Geometry: final body of the model. Coordinates: model frame, mm. A direction names the side the tool comes from. Give positions to 0.01 mm unless a question says otherwise; leave off trailing zeros. Order: outer loops, then holes, each group sorted by start corner. A loop starts at its lowest first (then second) coordinate and runs counter-clockwise, first axis right, second up. Notation, with made-up numbers: (-27.75, 49.5) - (16.25, 49.5) arc R9 ccw to (16.25, 61.5) - close; hole circle Ø8 at (8.5, 82.25). An arc over 180 degrees is marked (long way). One line per item, written item: value.
```python
from build123d import *

# Parameters (mm, degrees)
SKETCH1_R                     = 2.15265
SKETCH1_R_2                   = 9.525
BOSS_EXTRUDE1_DEPTH           = 1.5875
CUT_EXTRUDE1_DEPTH            = 2.54
F_13_64_0_18_DIAMETER_HOLE1_D = 4.572


with BuildPart() as part:
    # Sketch1 → Boss-Extrude1 (new body)
    with BuildSketch(Plane(origin=(0, 0, 0), x_dir=(1, 0, 0), z_dir=(0, 1, 0))):
        with BuildLine():
            Line((-107.315, 152.4), (-146.05, 152.4))
            Line((-146.05, 152.4), (-146.05, -152.4))
            Line((-146.05, -152.4), (146.05, -152.4))
            Line((146.05, -152.4), (146.05, 152.4))
            Line((146.05, 152.4), (107.315, 152.4))
            Line((107.315, 152.4), (107.315, 149.225))
            ThreePointArc((107.315, 149.225), (105.455128061, 144.734871939), (100.965, 142.875))
            Line((100.965, 142.875), (-100.965, 142.875))
            ThreePointArc((-100.965, 142.875), (-105.455128061, 144.734871939), (-107.315, 149.225))
            Line((-107.315, 149.225), (-107.315, 152.4))
        make_face()
        with Locations(Location((-135.128, -118.872, 0), (0, 0, 270))):
            Circle(SKETCH1_R, mode=Mode.SUBTRACT)
        with Locations(Location((-91.44, -91.44, 0), (0, 0, 270))):
            Circle(SKETCH1_R_2, mode=Mode.SUBTRACT)
        with Locations(Location((-113.665, -57.15, 0), (0, 0, 270))):
            Circle(SKETCH1_R, mode=Mode.SUBTRACT)
        with Locations(Location((-113.665, -38.1, 0), (0, 0, 270))):
            Circle(SKETCH1_R, mode=Mode.SUBTRACT)
        with Locations(Location((-91.44, -47.244, 0), (0, 0, 270))):
            Circle(SKETCH1_R_2, mode=Mode.SUBTRACT)
        with Locations(Location((-91.44, -3.048, 0), (0, 0, 270))):
            Circle(SKETCH1_R_2, mode=Mode.SUBTRACT)
        with BuildLine():
            ThreePointArc((-100.965, -117.475), (-107.315, -111.125), (-100.965, -104.775))
            Line((-100.965, -104.775), (100.965, -104.775))
            ThreePointArc((100.965, -104.775), (107.315, -111.125), (100.965, -117.475))
            Line((100.965, -117.475), (-100.965, -117.475))
        make_face(mode=Mode.SUBTRACT)
        with Locations(Location((135.128, -118.872, 0), (0, 0, 270))):
            Circle(SKETCH1_R, mode=Mode.SUBTRACT)
        with Locations(Location((91.44, -91.44, 0), (0, 0, 270))):
            Circle(SKETCH1_R_2, mode=Mode.SUBTRACT)
        with Locations(Location((91.44, -47.244, 0), (0, 0, 270))):
            Circle(SKETCH1_R_2, mode=Mode.SUBTRACT)
        with Locations(Location((113.665, -57.15, 0), (0, 0, 270))):
            Circle(SKETCH1_R, mode=Mode.SUBTRACT)
        with Locations(Location((113.665, -38.1, 0), (0, 0, 270))):
            Circle(SKETCH1_R, mode=Mode.SUBTRACT)
        with Locations(Location((91.44, -3.048, 0), (0, 0, 270))):
            Circle(SKETCH1_R_2, mode=Mode.SUBTRACT)
        with Locations(Location((-113.665, 76.2, 0), (0, 0, 270))):
            Circle(SKETCH1_R, mode=Mode.SUBTRACT)
        with Locations(Location((-91.44, 41.148, 0), (0, 0, 270))):
            Circle(SKETCH1_R_2, mode=Mode.SUBTRACT)
        with Locations(Location((-113.665, 95.25, 0), (0, 0, 270))):
            Circle(SKETCH1_R, mode=Mode.SUBTRACT)
        with Locations(Location((-91.44, 85.344, 0), (0, 0, 270))):
            Circle(SKETCH1_R_2, mode=Mode.SUBTRACT)
        with Locations(Location((-135.128, 141.478, 0), (0, 0, 270))):
            Circle(SKETCH1_R, mode=Mode.SUBTRACT)
        with Locations(Location((-91.44, 129.54, 0), (0, 0, 270))):
            Circle(SKETCH1_R_2, mode=Mode.SUBTRACT)
        with Locations(Location((91.44, 41.148, 0), (0, 0, 270))):
            Circle(SKETCH1_R_2, mode=Mode.SUBTRACT)
        with Locations(Location((113.665, 76.2, 0), (0, 0, 270))):
            Circle(SKETCH1_R, mode=Mode.SUBTRACT)
        with Locations(Location((91.44, 85.344, 0), (0, 0, 270))):
            Circle(SKETCH1_R_2, mode=Mode.SUBTRACT)
        with Locations(Location((113.665, 95.25, 0), (0, 0, 270))):
            Circle(SKETCH1_R, mode=Mode.SUBTRACT)
        with Locations(Location((91.44, 129.54, 0), (0, 0, 270))):
            Circle(SKETCH1_R_2, mode=Mode.SUBTRACT)
        with Locations(Location((135.128, 141.478, 0), (0, 0, 270))):
            Circle(SKETCH1_R, mode=Mode.SUBTRACT)
    extrude(amount=BOSS_EXTRUDE1_DEPTH)

    # Sketch2 → Cut-Extrude1 (cut)
    with BuildSketch(Plane(origin=(0, 1.5875, 0), x_dir=(1, 0, 0), z_dir=(0, 1, 0))):
        Polygon((-23.413358533, 142.875), (-29.763358533, 142.875), (-29.763358533, 116.18638997), (-29.763358533, 111.10638997), (-23.413358533, 111.10638997), (-10.745128401, 111.10638997), (-10.745128401, 80.773994761), (-10.745128401, 71.647772826), (-39.37, 71.647772826), (-39.37, 54.61788987), (-39.37, 43.18), (-33.02, 43.18), (-33.02, 54.61788987), (-33.02, 65.297772826), (-4.395128401, 65.297772826), (-4.395128401, 74.423994761), (-4.395128401, 82.043994761), (-4.395128401, 111.10638997), (-4.395128401, 117.45638997), (-23.413358533, 117.45638997), align=None)
        Polygon((51.818643407, 142.875), (45.468643407, 142.875), (45.468643407, 123.598152459), (26.196923788, 123.598152459), (26.196923788, 117.248152459), (26.196923788, 65.497956958), (50.548643407, 65.497956958), (50.548643407, 46.447956958), (26.196923788, 46.447956958), (25.908, -26.035), (32.258, -26.035), (32.258, -6.148708856), (32.258, -3.919741149), (32.258, 40.097956958), (56.898643407, 40.097956958), (56.898643407, 71.847956958), (32.546923788, 71.847956958), (32.546923788, 117.248152459), (51.818643407, 117.248152459), align=None)
    extrude(amount=-CUT_EXTRUDE1_DEPTH, mode=Mode.SUBTRACT)

    # 13/64 (0.18) Diameter Hole1 (through all)
    with Locations(Plane(origin=(0, 0, 0), x_dir=(-1, 0, 0), z_dir=(0, -1, 0))):
        with Locations((-57.15, 107.315), (-57.15, 84.455), (38.1, 84.455), (38.1, 107.315)):
            Hole(F_13_64_0_18_DIAMETER_HOLE1_D / 2)


solid = part.part
```
1) Mould query, pull axis Z, two halves, no side actions, for faces 4 (the face through (-2, 1.588, -2)), 5 (the face through (105.5, 0.78, -144.78)), 6 (the face through (107.313, 0.783, 110.985)). Classes: released by +Z, released by -Z, zero draft, split by the parting line, or undercut.
Answers below:
face 4: zero draft
face 5: released by -Z
face 6: undercut
2) Section A-A, the plane x = 17. Return loops of the section in (y, z) (1 decimal).
Answers below:
outline: (0, -142.9) - (1.6, -142.9) - (1.6, 104.8) - (0, 104.8) - close; (0, 117.5) - (1.6, 117.5) - (1.6, 152.4) - (0, 152.4) - close
3) First-contact query: pin 1 (0.8 mm diameter, centred on x = -81, y = 1, fed in from -Z) (3 decimals). Flat tip, straight axial feed; report the tip coordinate or a pass-through.
Answers below:
pin 1: z = -142.875
4) Material intervals for line 1 along Z through (x, y) = (-26, 0.5) (3 decimals); line 2 along X through (y, z) = (0.4, -61); line 3 along Z through (x, y) = (34, 1.55) (3 decimals), sorted ascending.
Answers below:
line 1: -111.106 to -71.648, -65.298 to 104.775, 117.475 to 152.4
line 2: -146.05 to -39.37, -33.02 to 50.55, 56.9 to 146.05
line 3: -142.875 to -123.598, -117.248 to -71.848, -65.498 to -46.448, -40.098 to 104.775, 117.475 to 152.4
5) Set-up query: faces 1 (the face through (-107.313, 0.783, 111.265)), 2 (the face through (-105.41, 0.78, -144.69)), 3 (the face through (-2, 0, -2)). Return all of +Z, -Z, +X, -X, +Y, -Y with unobstructed straight access to the full face (end or side cutting, diameter ignored); none if empty.
Answers below:
face 1: +Y, -Y
face 2: -Z, +Y, -Y
face 3: +Z, -Z, +X, -X, -Y
6) Section B-B, the plane z = 91.44. Count the separate pieces of the cut face and the enclosed holes in it, then the cut area to 3 significant figures.
Answers below:
separate pieces: 3
enclosed holes: 0
area: 403 mm^2
